Input: dimensioned drawing with shaded views. Units: mm. Origin: part minimum x, y, z. Give positions to 0.01 mm unless a question says otherwise; leave off trailing zeros. Write each loop counter-clockwise with the first axis right and the second up, starting at its lowest first coordinate (ties: lowest second). Pieces come first, ordered by that corner, then holes. Notation, with made-up numbers: (79, 77) - (102, 77) arc R24 cw to (102, 92) - close; hole circle Ø11 at (-38.75, 56). An arc over 180 degrees is marked (long way). Answer as a JSON object with one key per item and string values. Group by question number.
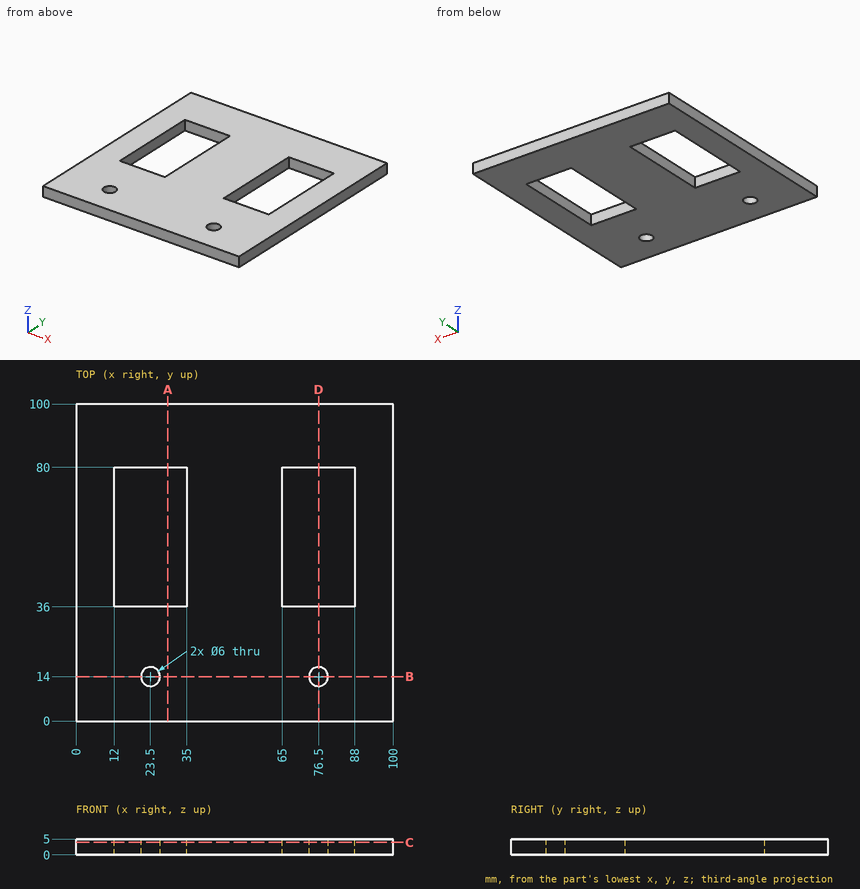
Q1. Section C-C on z = 3.95. Return the cut outline in (x, y), then the cut area to 3 significant figures.
Q2. Ray query, probe 1 along Y at (x, z) = (23.5, 3.35); probe 2 along X at (y, z) = (71.5, 4.85); probe 3 along Y at (x, z) = (83, 2.25). Return the intervals inside material, ascending. Write a range as [from, to].
Q3. Section A-A on x = 29. Return the cut outline in (y, z), then the cut area to 3 significant figures.
Q4. Section B-B on y = 14. Return the cut outline in (x, z), then the cut area to 3 significant figures.
Q5. Section D-D on x = 76.5. Return the cut outline in (y, z).
Taken from the geometry:
{
 "1": {"outline": "(0, 0) - (100, 0) - (100, 100) - (0, 100) - close; hole (12, 36) - (35, 36) - (35, 80) - (12, 80) - close; hole circle Ø6 at (23.5, 14); hole (65, 36) - (88, 36) - (88, 80) - (65, 80) - close; hole circle Ø6 at (76.5, 14)", "area": "7,920 mm²"},
 "2": {"probe 1": "y = [0, 11], [17, 36], [80, 100]", "probe 2": "x = [0, 12], [35, 65], [88, 100]", "probe 3": "y = [0, 36], [80, 100]"},
 "3": {"outline": "(0, 0) - (36, 0) - (36, 5) - (0, 5) - close; (80, 0) - (100, 0) - (100, 5) - (80, 5) - close", "area": "280 mm²"},
 "4": {"outline": "(0, 0) - (20.5, 0) - (20.5, 5) - (0, 5) - close; (26.5, 0) - (73.5, 0) - (73.5, 5) - (26.5, 5) - close; (79.5, 0) - (100, 0) - (100, 5) - (79.5, 5) - close", "area": "440 mm²"},
 "5": {"outline": "(0, 0) - (11, 0) - (11, 5) - (0, 5) - close; (17, 0) - (36, 0) - (36, 5) - (17, 5) - close; (80, 0) - (100, 0) - (100, 5) - (80, 5) - close"}
}
